Design review of the part shown in the three views and the two pictorial views. Dimensions are in mm from the part's minimum x, y and z. Coordinates: 2 decimals unless noted, no trailing zeros. Write each loop counter-clockwise with the first axis right and the second up, starting at its lowest first coordinate (ties: lowest second). Pieces come first, ordered by that corner, then holes. Notation, with made-up numbers: (60, 2) -> (68, 2) arc R32 ccw to (68, 32) -> close; hole circle Ø7 at (-29, 74.25). An arc over 180 degrees is marked (long way). Write each question's results on one line, items separated by ' | '.
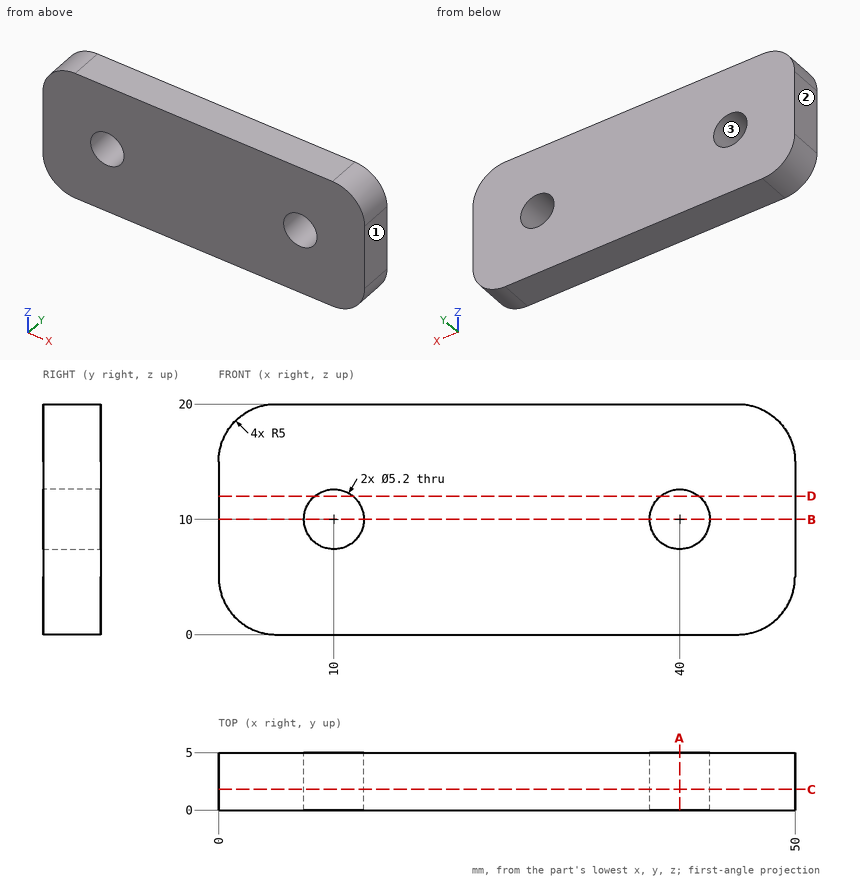
Q1. Add section D-D (z = 12). Write out the cut boundary in (x, y), plus the area to 3 significant figures.
Solution:
outline: (0, 0) -> (8.34, 0) -> (8.34, 5) -> (0, 5) -> close; (11.66, 0) -> (38.34, 0) -> (38.34, 5) -> (11.66, 5) -> close; (41.66, 0) -> (50, 0) -> (50, 5) -> (41.66, 5) -> close | area: 217 mm²
Q2. Add section B-B (z = 10). Write out the cut boundary in (x, y), plus the area to 3 significant figures.
Solution:
outline: (0, 0) -> (7.4, 0) -> (7.4, 5) -> (0, 5) -> close; (12.6, 0) -> (37.4, 0) -> (37.4, 5) -> (12.6, 5) -> close; (42.6, 0) -> (50, 0) -> (50, 5) -> (42.6, 5) -> close | area: 198 mm²
Q3. For line 1 (X direction, y = 2.8, z = 10); line 2 (X direction, y = 3, z = 12); line 3 (Z direction, x = 39.5, y = 2.95), list the stretches that pass through material, from the lowest coordinate up. Write a range as from..to.
Solution:
line 1: 0..7.4, 12.6..37.4, 42.6..50 | line 2: 0..8.34, 11.66..38.34, 41.66..50 | line 3: 0..7.45, 12.55..20
Q4. Add section A-A (x = 40). Write out the cut boundary in (y, z), plus the area to 3 significant figures.
Solution:
outline: (0, 0) -> (5, 0) -> (5, 7.4) -> (0, 7.4) -> close; (0, 12.6) -> (5, 12.6) -> (5, 20) -> (0, 20) -> close | area: 74.0 mm²
Q5. Add section C-C (y = 1.8). Write out the cut boundary in (x, z).
Solution:
outline: (0, 5) arc R5 ccw to (5, 0) -> (45, 0) arc R5 ccw to (50, 5) -> (50, 15) arc R5 ccw to (45, 20) -> (5, 20) arc R5 ccw to (0, 15) -> close; hole circle Ø5.2 at (10, 10); hole circle Ø5.2 at (40, 10)
Q6. Clearance check with a flat-ended pin moving along its axis: P1, Ø3, axis at x = 10, z = 10, coming from the +Y side. State where the tip first meets the part, or that it passes through.
Solution:
P1: through
Q7. Draft analysis for pull direction X (two halves, no side actions). For the marked faces 1, 2 and 3, state which applies: pulls with the +X half, pulls with the -X half, needs draft (parallel to the pull), parting line crosses it, or undercut.
Solution:
face 1: pulls with the +X half | face 2: pulls with the -X half | face 3: undercut
